```python
from build123d import *

# Parameters (mm, degrees)
F0_W     = 127
F0_H     = 76.2
F1_DEPTH = 25.4
F2_R     = 6.35
F3_DEPTH = 25.4
F4_W     = 25.4
F4_H     = 50.8
F6_W     = 50.640457
F6_H     = 23.190491


with BuildPart() as f1:
    # F0 (on Top) → F1 (new body)
    with BuildSketch(Plane.XY):
        Rectangle(F0_W, F0_H)
    extrude(amount=F1_DEPTH)

    # F2 (on face) → F3 (cut)
    with BuildSketch(Plane.XY.offset(25.4)):
        with Locations((50.8, -25.4)):
            Circle(F2_R)
        with Locations((-50.8, -25.4)):
            Circle(F2_R)
        with Locations((50.8, 25.4)):
            Circle(F2_R)
        with Locations((-50.8, 25.4)):
            Circle(F2_R)
    extrude(amount=-F3_DEPTH, mode=Mode.SUBTRACT)

    # F4 (on Front) → F5 (revolve)
    with BuildSketch(Plane.XZ):
        with Locations((-12.7, 50.8)):
            Rectangle(F4_W, F4_H)
    revolve(axis=Axis((0, 0, 50.8), (0, 0, 1)))

    # F6 (on Front) → F7 (revolve, cut)
    with BuildSketch(Plane.XZ):
        with Locations((34.864176, 43.432057)):
            Rectangle(F6_W, F6_H)
    revolve(axis=Axis((0, 0, 76.2), (0, 0, -1)), mode=Mode.SUBTRACT)


solid = f1.part
```
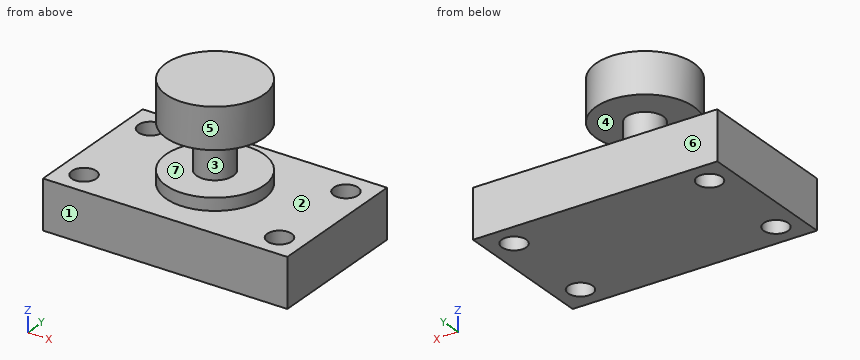
Source: CAD feature listing. Evaluate the final solid. Frame: model axes, mm. Face numbers are marked on the shaded views. A direction names the side the tool comes from. Round coordinates to 2 decimals unless told otherwise and drop trailing zeros. Loops run counter-clockwise (first coordinate to the right, second up) from the corner with the lowest first, then second, coordinate; pieces in that order, holes last.
1. Ray query, L1, parallel to Y at x = 50.8, z = 11.5; L2, parallel to Z at x = -8, y = -16.5; L3, parallel to Y at x = -52.5, z = 15. Return the intervals inside material, ascending.
2. Access query for the marked faces 5, 6 and 7. Directions: +Z, -Z, +X, -X, +Y, -Y. A direction counts if a zero-diameter tool reaches every point of the face in a straight line with its end or side. Return the directions, or none.
3. Section query D-D on y = 0. Output: boundary loops of the cut face in (x, z), and give its area (3 significant figures).
4. Section query C-C on y = 20.5. Output: boundary loops of the cut face in (x, z).
5. Mould query, pull axis Z, two halves, no side actions, for the marked faces 1, 2, 3 and 4. Classes: released by +Z, released by -Z, zero draft, split by the parting line, or undercut.
6. Section query A-A on z = 18. Output: boundary loops of the cut face in (x, y).
7. Contact query for flat-ended pins moving along their axis: pin 1 (10 mm diameter, centred on x = -32.5, y = 30.5, fed in from +Z); pin 2 (12 mm diameter, centred on y = -3, z = 34.5, fed in from +X). Output: stop coordinate, or through.
8. Section query B-B on x = 50.8. Output: boundary loops of the cut face in (y, z).
Answers below:
1. L1: y = -38.1 to -31.75, -19.05 to 19.05, 31.75 to 38.1
1. L2: z = 0 to 31.84, 55.03 to 76.2
1. L3: y = -38.1 to -31.52, -19.28 to 19.28, 31.52 to 38.1
2. face 5: +Z
2. face 6: +Z, -Z, +X, -X, +Y
2. face 7: none
3. outline: (-63.5, 0) - (63.5, 0) - (63.5, 25.4) - (25.4, 25.4) - (25.4, 31.84) - (9.54, 31.84) - (9.54, 55.03) - (25.4, 55.03) - (25.4, 76.2) - (-25.4, 76.2) - (-25.4, 55.03) - (-9.54, 55.03) - (-9.54, 31.84) - (-25.4, 31.84) - (-25.4, 25.4) - (-63.5, 25.4) - close
3. area: 5,070 mm2
4. outline: (-63.5, 0) - (-54.84, 0) - (-54.84, 25.4) - (-63.5, 25.4) - close; (-46.76, 0) - (46.76, 0) - (46.76, 25.4) - (15, 25.4) - (15, 31.84) - (-15, 31.84) - (-15, 25.4) - (-46.76, 25.4) - close; (-15, 55.03) - (15, 55.03) - (15, 76.2) - (-15, 76.2) - close; (54.84, 0) - (63.5, 0) - (63.5, 25.4) - (54.84, 25.4) - close
5. face 1: zero draft
5. face 2: released by +Z
5. face 3: undercut
5. face 4: undercut
6. outline: (-63.5, -38.1) - (63.5, -38.1) - (63.5, 38.1) - (-63.5, 38.1) - close; hole circle Ø12.7 at (-50.8, -25.4); hole circle Ø12.7 at (-50.8, 25.4); hole circle Ø12.7 at (50.8, -25.4); hole circle Ø12.7 at (50.8, 25.4)
7. pin 1: stops at z = 25.4
7. pin 2: stops at x = 25.4
8. outline: (-38.1, 0) - (-31.75, 0) - (-31.75, 25.4) - (-38.1, 25.4) - close; (-19.05, 0) - (19.05, 0) - (19.05, 25.4) - (-19.05, 25.4) - close; (31.75, 0) - (38.1, 0) - (38.1, 25.4) - (31.75, 25.4) - close
